Verification items for the finished model (mm, model axes). A direction names the side the tool comes from. Coordinates: 2 decimals unless noted, no trailing zeros. Write each loop counter-clockwise with the first axis right and the second up, starting at its lowest first coordinate (ties: lowest second). Pieces come first, ordered by that corner, then holes. Notation, with made-up numbers: (-30.75, 64.25) - (-4.75, 64.25) arc R19 cw to (-4.75, 82.25) - close; hole circle Ø5 at (81, 42.5). An arc over 180 degrees is marked (long way). Use one line per item in the form item = value. Start each with the question number.
(1) Gauge pin test, flat ends, axial feed: pin 1 Ø1 at (x, z) = (0, 0) entering from +Y; pin 2 Ø1.5 at (x, z) = (0, 0) entering from -Y. Record the tip position at first contact, or that the pin passes through.
(2) Sectioned sample at B-B (y = -8.5). Record the cut outline in (x, z), and give its area (3 significant figures).
(3) Material ranges on line 1 (X direction, y = -28.3, z = 0) (3 decimals); line 2 (Y direction, x = 0, z = -0.6); line 3 (Z direction, x = 1.85, y = 21.5), recorded low to high. Write a range as [from, to].
(4) Sectioned sample at A-A (x = 0). Record the cut outline in (y, z) (3 decimals).
(5) Mould release check, pull along Z, two halves, no side actions. Record for faces 3 (the flat face through (0, -26.15, 0)), 4 (the cylindrical face through (-2.5, 0.4, -0.1)), 5 (the cylindrical face through (-0.502, -28.685, -0.655)), 6 (the flat face through (-1, 31.15, 0)): released by +Z, released by -Z, zero draft, split by the parting line, or undercut.
(6) Tool access check on faces 1 (the flat face through (2, 0, 0)), 2 (the cylindrical face through (-0.502, 28.685, -0.655)). Record the directions out of +Z, -Z, +X, -X, +Y, -Y that give a thin tool (end or side, any length) a straight path to the whole face; none if there is none.
from build123d import *

# Parameters (mm, degrees)
SKETCH1_R            = 2.5
BOSS_EXTRUDE1_DEPTH  = 31.15
SKETCH2_R            = 0.825
CUT_EXTRUDE1_DEPTH   = 5
CUT_EXTRUDE2_DEPTH   = 32.35
FILLET1_R            = 0.5
FILLET1_OF_MIRROR1_R = 0.5


with BuildPart() as part:
    # Sketch1 → Boss-Extrude1 (new body)
    with BuildSketch(Plane(origin=(0, 0, 0), x_dir=(1, 0, 0), z_dir=(0, 1, 0))):
        with Locations(Location((0, 0, 0), (0, 0, 270))):
            Circle(SKETCH1_R)
    boss_extrude1 = extrude(amount=BOSS_EXTRUDE1_DEPTH)

    # Sketch2 → Cut-Extrude1 (cut)
    with BuildSketch(Plane(origin=(0, 31.15, 0), x_dir=(1, 0, 0), z_dir=(0, 1, 0))):
        with Locations(Location((0, 0, 0), (0, 0, 270))):
            Circle(SKETCH2_R)
    cut_extrude1 = extrude(amount=-CUT_EXTRUDE1_DEPTH, mode=Mode.SUBTRACT)

    # Sketch3 → Cut-Extrude2 (cut, through all)
    with BuildSketch(Plane(origin=(0, 31.15, 0), x_dir=(1, 0, 0), z_dir=(0, 1, 0))):
        with BuildLine():
            Line((2, 1.5), (2, -1.5))
            ThreePointArc((2, -1.5), (2.5, 0), (2, 1.5))
        make_face()
    cut_extrude2 = extrude(amount=-CUT_EXTRUDE2_DEPTH, mode=Mode.SUBTRACT)

    # Fillet1
    fillet1_edges = [part.edges().sort_by_distance(p)[0] for p in [
        (-2.5, 31.15, 0),
    ]]
    fillet(fillet1_edges, radius=FILLET1_R - 0.0001)  # a hair under: the kernel refuses the full size

    # Mirror1: Boss-Extrude1, Cut-Extrude1, Cut-Extrude2 across plane
    add(boss_extrude1.mirror(Plane.ZX))
    add(cut_extrude1.mirror(Plane.ZX), mode=Mode.SUBTRACT)
    add(cut_extrude2.mirror(Plane.ZX), mode=Mode.SUBTRACT)

    # Fillet1 of Mirror1
    fillet1_of_mirror1_edges = [part.edges().sort_by_distance(p)[0] for p in [
        (-2.5, -31.15, 0),
    ]]
    fillet(fillet1_of_mirror1_edges, radius=FILLET1_OF_MIRROR1_R - 0.0001)  # a hair under: the kernel refuses the full size


solid = part.part
Answers below:
q1.pin_1 = 26.15
q1.pin_2 = -26.15
q2.outline = (2, -1.5) - (2, 1.5) arc R2.5 ccw (long way) to start
q2.area = 18.6 mm2
q3.line_1 = [-2.5, -0.825], [0.825, 2]
q3.line_2 = [-26.15, 26.15]
q3.line_3 = [-1.68, 1.68]
q4.outline = (-31.15, -2) arc R0.5 ccw to (-30.65, -2.5) - (30.65, -2.5) arc R0.5 ccw to (31.15, -2) - (31.15, -0.825) - (26.15, -0.825) - (26.15, 0.825) - (31.15, 0.825) - (31.15, 2) arc R0.5 ccw to (30.65, 2.5) - (-30.65, 2.5) arc R0.5 ccw to (-31.15, 2) - (-31.15, 0.825) - (-26.15, 0.825) - (-26.15, -0.825) - (-31.15, -0.825) - close
q5.face_3 = undercut
q5.face_4 = split by the parting line
q5.face_5 = undercut
q5.face_6 = zero draft
q6.face_1 = +Z, -Z, +X, +Y, -Y
q6.face_2 = +Y
